Read the model definition and answer for the solid it produces. Units are mm, in the model's axes. A direction names the side the tool comes from. Give positions to 0.01 mm unless a question says otherwise; leave off trailing zeros. Order: outer loops, then holes, each group sorted by start corner. A loop starts at its lowest first (then second) coordinate and runs counter-clockwise, first axis right, second up. Notation, with made-up numbers: M 49,22.25 L 61,22.25 A16 cw 61,34.25 Z; hole C 88.25,42 d5. An arc over 180 degrees is marked long. One line per item, written item: value.
from build123d import *

# Parameters (mm, degrees)
SKETCH1_R               = 5
SKETCH1_R_2             = 2.25
BOSS_EXTRUDE1_DEPTH     = 50
CUT_EXTRUDE1_DEPTH      = 52
CUT_EXTRUDE1_DEPTH_BACK = 35
SKETCH2_W               = 30
SKETCH2_H               = 60
SKETCH3_W               = 30
SKETCH3_H               = 40
CUT_EXTRUDE2_DEPTH      = 52
CUT_EXTRUDE3_START      = -10
CUT_EXTRUDE3_DEPTH      = 30
CUT_EXTRUDE4_START      = -10
CUT_EXTRUDE4_DEPTH      = 30
BOSS_EXTRUDE2_DEPTH     = 50
SKETCH8_R               = 2
CUT_EXTRUDE5_DEPTH      = 10
FILLET1_R               = 10


with BuildPart() as part:
    # Sketch1 → Boss-Extrude1 (new body)
    with BuildSketch(Plane(origin=(0, 0, 0), x_dir=(0, 0, -1), z_dir=(1, 0, 0))):
        with BuildLine():
            Line((-255.87149894, 42.046001407), (44.12850106, 42.046001407))
            add(Edge.make_bspline(
                [(44.12850106, 42.046001407), (124.12850106, 17.046001407), (44.12850106, -7.953998593)],
                knots=[0, 0, 0, 1, 1, 1], degree=2))
            Line((44.12850106, -7.953998593), (-255.87149894, -7.953998593))
            add(Edge.make_bspline(
                [(-255.87149894, 42.046001407), (-335.87149894, 17.046001407), (-255.87149894, -7.953998593)],
                knots=[0, 0, 0, 1, 1, 1], degree=2))
        make_face()
        with Locations((-280.87149894, 17.046001407)):
            Circle(SKETCH1_R, mode=Mode.SUBTRACT)
        with Locations((69.12850106, 17.046001407)):
            Circle(SKETCH1_R_2, mode=Mode.SUBTRACT)
    extrude(amount=BOSS_EXTRUDE1_DEPTH)

    # Sketch2 → Cut-Extrude1 (cut, two sides: drawn at the far end of the back side and taken through both)
    with BuildSketch(Plane(origin=(0, 0, 0), x_dir=(1, 0, 0), z_dir=(0, 1, 0)).offset(-CUT_EXTRUDE1_DEPTH_BACK)):
        with Locations((25, 54.12850106)):
            Rectangle(SKETCH2_W, SKETCH2_H)
    extrude(amount=CUT_EXTRUDE1_DEPTH + CUT_EXTRUDE1_DEPTH_BACK, mode=Mode.SUBTRACT)

    # Sketch3 → Cut-Extrude2 (cut)
    with BuildSketch(Plane.XZ.offset(7.953998593)):
        with Locations((25, 275.87149894)):
            Rectangle(SKETCH3_W, SKETCH3_H)
    extrude(amount=-CUT_EXTRUDE2_DEPTH, mode=Mode.SUBTRACT)

    # Sketch4 → Cut-Extrude3 (cut)
    with BuildSketch(Plane.ZY.offset(CUT_EXTRUDE3_START)):
        Polygon((-24.12850106, 17.046001407), (-24.12850106, 42.046001407), (19.172769129, 42.046001407), align=None)
    extrude(amount=-CUT_EXTRUDE3_DEPTH, mode=Mode.SUBTRACT)

    # Sketch5 → Cut-Extrude4 (cut)
    with BuildSketch(Plane.ZY.offset(CUT_EXTRUDE4_START)):
        Polygon((-24.12850106, -7.953998593), (-24.12850106, 17.046001407), (19.172769129, -7.953998593), align=None)
    extrude(amount=-CUT_EXTRUDE4_DEPTH, mode=Mode.SUBTRACT)

    # Sketch6 → Boss-Extrude2 (add)
    with BuildSketch(Plane(origin=(0, 42.046001407, 0), x_dir=(1, 0, 0), z_dir=(0, 1, 0))):
        Polygon((50, -35.87149894), (85, -35.87149894), (85, 84.12850106), (80, 84.12850106), (80, -15.87149894), (50, -15.87149894), align=None)
    extrude(amount=-BOSS_EXTRUDE2_DEPTH)

    # Sketch8 → Cut-Extrude5 (cut)
    with BuildSketch(Plane(origin=(85, 0, 0), x_dir=(0, 0, -1), z_dir=(1, 0, 0))):
        with Locations((14.12850106, 29.546001407)):
            Circle(SKETCH8_R)
        with Locations((26.62850106, 17.046001407)):
            Circle(SKETCH8_R)
        with Locations((14.12850106, 4.546001407)):
            Circle(SKETCH8_R)
        with Locations((1.62850106, 17.046001407)):
            Circle(SKETCH8_R)
    extrude(amount=-CUT_EXTRUDE5_DEPTH, mode=Mode.SUBTRACT)

    # Fillet1
    fillet1_edges = [part.edges().sort_by_distance(p)[0] for p in [
        (25, 17.046001407, -24.12850106),
    ]]
    fillet(fillet1_edges, radius=FILLET1_R)


solid = part.part
1) Find section B-B, the plane x = 18. Write down the section's boundary in (y, z), plus the area to 3 significant figures.
Reported:
outline: M -7.95,19.17 L 8.39,-9.13 A10 ccw 25.71,-9.13 L 42.05,19.17 L 42.05,255.87 L -7.95,255.87 Z
area: 12,800 mm^2
2) Find section C-C, the plane z = 245.5. Write down the section's boundary in (x, y).
Reported:
outline: M 0,-7.95 L 50,-7.95 L 50,42.05 L 0,42.05 Z
3) Find section A-A, the plane z = -36. Write down the section's boundary in (x, y).
Reported:
outline: M 0,-7.95 L 10,-7.95 L 10,42.05 L 0,42.05 Z; M 40,-7.95 L 50,-7.95 L 50,42.05 L 40,42.05 Z; M 80,-7.95 L 85,-7.95 L 85,42.05 L 80,42.05 Z
4) Find section D-D, the plane x = 68. Write down the section's boundary in (y, z).
Reported:
outline: M -7.95,15.87 L 42.05,15.87 L 42.05,35.87 L -7.95,35.87 Z
5) Determine the mould class of faces 6 (the face through (4.93, 17.266, 285.867)), 7 (the face through (44.93, 17.266, 285.867)), 8 (the face through (24.79, 33.99, 5.22)), 9 (the face through (10, 17, -32)) for opening direction Y: +Y half, -Y half, draft (parallel to the pull), parting line (faces both ways), or undercut.
Reported:
face 6: undercut
face 7: undercut
face 8: +Y half
face 9: draft
6) Consider probe 1 along X at (y, z) = (23.5, -32); probe 2 along X at (y, z) = (17, -27.5); probe 3 along X at (y, z) = (12.5, 11.5). Determine where each line is inside the solid, lowest interval first.
Reported:
probe 1: x = 0 to 10, 40 to 50, 80 to 85
probe 2: x = 0 to 10, 40 to 50
probe 3: x = 0 to 50, 80 to 85
7) Which of the six approach directions +Z, -Z, +X, -X, +Y, -Y give full straight-line access (tool end or side, diameter ignored) to faces 1 (the face through (25.21, 17.193, -14.127)), 2 (the face through (50, 17, 150)), 3 (the face through (24.79, 0.33, 4.824)), 4 (the face through (65, 17, 15.871)), 5 (the face through (40, 17, 271))?
Reported:
face 1: -Z
face 2: +Z, +X, +Y, -Y
face 3: -Z, -Y
face 4: -Z, +Y, -Y
face 5: +Z, +Y, -Y
8) Each of these flat-tipped pins is pushed along its axis until it touches: pin 1 Ø3.5 at (y, z) = (17.05, -26.63) entering from +X; pin 2 Ø5 at (x, y) = (11.5, 34.5) entering from -Z; pin 3 Ø3 at (x, y) = (18.5, 2.5) entering from -Z. Where does it stop, or does it pass through?
Reported:
pin 1: stops at x = 50
pin 2: stops at z = -68.84
pin 3: stops at z = -1.53
